from build123d import *

# Parameters (mm, degrees)
F0_W     = 38.1
F0_H     = 25.4
F1_DEPTH = 57.15
F3_DEPTH = 38.101
F5_DEPTH = 12.7
F7_DEPTH = 12.7


with BuildPart() as f1:
    # F0 (on Right) → F1 (new body)
    with BuildSketch(Plane.YZ):
        with Locations((2.271346, 12.7)):
            Rectangle(F0_W, F0_H)
    extrude(amount=F1_DEPTH)

    # F2 (on face) → F3 (cut, through all)
    with BuildSketch(Plane.XZ.offset(16.778654)):
        Polygon((44.45, 25.4), (57.15, 0), (57.15, 25.4), align=None)
    extrude(amount=-F3_DEPTH, mode=Mode.SUBTRACT)

    # F4 (on face) → F5 (cut)
    with BuildSketch(Plane.XZ.offset(16.778654)):
        Polygon((44.45, 25.4), (19.065139, 25.4), (31.75, 0), (57.15, 0), align=None)
    extrude(amount=-F5_DEPTH, mode=Mode.SUBTRACT)

    # F6 (on face) → F7 (cut)
    with BuildSketch(Plane(origin=(0, 21.321346, 0), x_dir=(-1, 0, 0), z_dir=(0, 1, 0))):
        Polygon((-57.15, 0), (-31.75, 0), (-22.225, 25.4), (-44.45, 25.4), align=None)
    extrude(amount=-F7_DEPTH, mode=Mode.SUBTRACT)


solid = f1.part
Could you check a few things on this model? Use its own coordinates, in mm. A direction names the side the tool comes from. Coordinates: 2 decimals unless noted, no trailing zeros. Loops run counter-clockwise (first coordinate to the right, second up) from the corner with the lowest first, then second, coordinate; pieces in that order, holes last.
1. Imagine slicing it at C-C (x = 27). Please give me the cut outline in (y, z), and give its area (3 significant figures).
2. Imagine slicing it at D-D (y = -5). Please give me the cut outline in (x, z).
3. Imagine slicing it at A-A (z = 23.75). Please give me the cut outline in (x, y) (3 decimals).
4. For P1, Ø8, axis at x = 46, z = 16, coming from the +Y side; P2, Ø5, axis at x = 24, y = 3, coming from the -Z side, each with a flat end and sliding along its axis, tell me the tip position at first contact or that it passes through.
5. Imagine slicing it at B-B (y = 4). Please give me the cut outline in (x, z).
6. For faces 1 (the face through (25.319, -10.518, 12.878)), 2 (the face through (40, 8.621, 13)), 3 (the face through (0, 2, 13)), which set-ups out of +Z, -Z, +X, -X, +Y, -Y let a thin tool reach every point of the face, with its end or its side?
7. I need wall thicknesses on L1, parallel to Y at x = 41, z = 2; L2, parallel to X at y = -1, z = 14.5; L3, parallel to X at y = -11, z = 14. Which ranges of each line are inside material? Lowest first, please.
Computed values:
1. outline: (-16.78, 0) - (21.32, 0) - (21.32, 12.67) - (8.62, 12.67) - (8.62, 25.4) - (-4.08, 25.4) - (-4.08, 9.51) - (-16.78, 9.51) - close
1. area: 604 mm2
2. outline: (0, 0) - (31.75, 0) - (19.07, 25.4) - (0, 25.4) - close
3. outline: (0, -16.779) - (19.889, -16.779) - (19.889, -4.079) - (45.275, -4.079) - (45.275, 8.621) - (22.844, 8.621) - (22.844, 21.321) - (0, 21.321) - close
4. P1: stops at y = 8.62
4. P2: stops at z = 0
5. outline: (0, 0) - (57.15, 0) - (44.45, 25.4) - (0, 25.4) - close
6. face 1: +Z, +X, -Y
6. face 2: +Z, +X, +Y
6. face 3: +Z, -Z, -X, +Y, -Y
7. L1: y = -4.08 to 8.62
7. L2: x = 0 to 49.9
7. L3: x = 0 to 24.76
